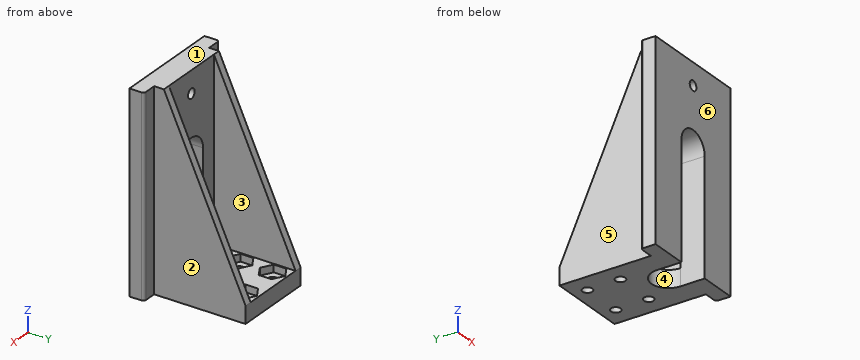
Autodesk Inventor part; units mm, degrees
ref_plane "YZ Plane" through (0, 0, 0) normal (1, 0, 0) x (0, 1, 0)
ref_plane "XZ Plane" through (0, 0, 0) normal (0, 1, 0) x (-1, 0, 0)
ref_plane "XY Plane" through (0, 0, 0) normal (0, 0, 1) x (1, 0, 0)
sketch "Sketch1" plane through (0, 0, 0) normal (0, 0, 1) x (1, 0, 0)
  line L0 (0, 43.4) -> (27, 43.4)
  line L1 (27, 43.4) -> (27, 0)
  line L2 (27, 0) -> (0, 0)
  line L3 (0, 0) -> (0, 43.4)
  circle A0 centre (5, 37.4) radius 2
  circle A1 centre (22, 37.4) radius 2
  circle A2 centre (5, 23.91) radius 2
  circle A3 centre (22, 23.91) radius 2
  dimension "d0" = 27
  dimension "d1" = 43.4
  dimension "d2" = 4
  dimension "d3" = 6
  dimension "d4" = 6
  dimension "d5" = 5
  dimension "d6" = 5
  dimension "d7" = 5
  dimension "d8" = 5
  dimension "d61" = 13.49
  dimension "d62" = 13.49
extrude "Extrusion1" add sketch "Sketch1" along normal blind 7
sketch "Sketch2" plane through (0, 0, 7) normal (0, 0, 1) x (1, 0, 0)
  line L0 (0, 10) -> (27, 10)
  line L1 (27, 10) -> (27, 0)
  line L2 (27, 0) -> (0, 0)
  line L3 (0, 0) -> (0, 10)
  line L4 (0, 0) -> (27, 0)
  line L5 (0, 43.4) -> (0, 0)
  line L6 (27, 0) -> (27, 43.4)
  dimension "d13" = 10
extrude "Extrusion2" add sketch "Sketch2" along normal blind 73
sketch "Sketch3" plane through (0, 0, 7) normal (0, 0, 1) x (1, 0, 0)
  line L0 (0.5, 39.9981) -> (0.5, 34.8019)
  line L1 (0.5, 34.8019) -> (5, 32.2038)
  line L2 (5, 32.2038) -> (9.5, 34.8019)
  line L3 (9.5, 34.8019) -> (9.5, 39.9981)
  line L4 (9.5, 39.9981) -> (5, 42.5962)
  line L5 (5, 42.5962) -> (0.5, 39.9981)
  circle A0 centre (5, 37.4) radius 4.5
  circle A1 centre (5, 37.4) radius 2
  line L6 (17.5, 39.9981) -> (17.5, 34.8019)
  line L7 (17.5, 34.8019) -> (22, 32.2038)
  line L8 (22, 32.2038) -> (26.5, 34.8019)
  line L9 (26.5, 34.8019) -> (26.5, 39.9981)
  line L10 (26.5, 39.9981) -> (22, 42.5962)
  line L11 (22, 42.5962) -> (17.5, 39.9981)
  circle A2 centre (22, 37.4) radius 4.5
  line L12 (17.5, 26.5081) -> (17.5, 21.3119)
  line L13 (17.5, 21.3119) -> (22, 18.7138)
  line L14 (22, 18.7138) -> (26.5, 21.3119)
  line L15 (26.5, 21.3119) -> (26.5, 26.5081)
  line L16 (26.5, 26.5081) -> (22, 29.1062)
  line L17 (22, 29.1062) -> (17.5, 26.5081)
  circle A3 centre (22, 23.91) radius 4.5
  line L18 (0.5, 26.5081) -> (0.5, 21.3119)
  line L19 (0.5, 21.3119) -> (5, 18.7138)
  line L20 (5, 18.7138) -> (9.5, 21.3119)
  line L21 (9.5, 21.3119) -> (9.5, 26.5081)
  line L22 (9.5, 26.5081) -> (5, 29.1062)
  line L23 (5, 29.1062) -> (0.5, 26.5081)
  circle A4 centre (5, 23.91) radius 4.5
  circle A5 centre (22, 37.4) radius 2
  circle A6 centre (22, 23.91) radius 2
  circle A7 centre (5, 23.91) radius 2
  point P0 (0, 0)
  dimension "d16" = 120
  dimension "d17" = 120
  dimension "d18" = 9
  dimension "d19" = 120
  dimension "d20" = 120
  dimension "d21" = 9
  dimension "d22" = 120
  dimension "d23" = 120
  dimension "d24" = 9
  dimension "d25" = 120
  dimension "d26" = 120
  dimension "d27" = 9
extrude "Extrusion3" cut sketch "Sketch3" against normal blind 3 contours L5 A0 L0 | A0 L1 L0 | A0 | L5 L4 A0 | A0 L2 L1 | L4 L3 A0 | A0 L3 L2 | A1 | L11 A2 L6 | A2 L7 L6 | A2 | L11 L10 A2 | A2 L8 L7 | L10 L9 A2 | A2 L9 L8 | L17 A3 L12 | A3 L13 L12 | A3 | L17 L16 A3 | A3 L14 L13 | L16 L15 A3 | A3 L15 L14 | L23 A4 L18 | A4 L19 L18 | A4 | L23 L22 A4 | A4 L20 L19 | L22 L21 A4 | A4 L21 L20 | A5 | A6 | A7
sketch "Sketch4" plane through (27, 0, 0) normal (1, 0, 0) x (0, 0, -1)
  line L0 (-80, 10) -> (-80, 0)
  line L1 (-7, 43.4) -> (-80, 10)
  line L2 (-80, 10) -> (-80, 0)
  line L3 (0, 43.4) -> (0, 0)
  line L4 (-80, 0) -> (0, 0)
  line L5 (0, 0) -> (0, 43.4)
  line L6 (0, 43.4) -> (-7, 43.4)
  line L7 (0, 43.4) -> (-7, 43.4)
extrude "Extrusion4" add sketch "Sketch4" along normal blind 3
sketch "Sketch5" plane through (0, 0, 0) normal (-1, 0, 0) x (0, 0, 1)
  line L0 (80, 0) -> (0, 0)
  line L1 (80, 10) -> (80, 0)
  line L2 (80, 0) -> (80, 10)
  line L3 (7, 43.4) -> (80, 10)
  line L4 (80, 10) -> (7, 43.4)
  line L5 (0, 43.4) -> (7, 43.4)
  line L6 (7, 43.4) -> (0, 43.4)
  line L7 (0, 43.4) -> (0, 0)
  line L8 (0, 43.4) -> (0, 0)
  line L9 (0, 0) -> (80, 0)
extrude "Extrusion5" add sketch "Sketch5" along normal blind 3
sketch "Sketch6" plane through (27, 10, 80) normal (0, 1, 0) x (1, 0, 0)
  circle A0 centre (-13.5, 9) radius 2
  line L0 (-27, 0) -> (-27, 73)
  line L1 (0, 0) -> (-27, 0)
  line L2 (-30, 80) -> (3, 80)
  point P0 (-27, 80)
  dimension "d34" = 4
  dimension "d35" = 13.5
  dimension "d45" = 71
extrude "Extrusion6" cut sketch "Sketch6" against normal blind 74
sketch "Sketch7" plane through (30, 0, 0) normal (0, -1, 0) x (1, 0, 0)
  line L0 (-9.5, 47) -> (-9.5, 0)
  line L1 (-9.5, 0) -> (-23.5, 0)
  line L2 (-23.5, 0) -> (-23.5, 47)
  line L3 (0, 80) -> (0, 0)
  line L4 (-33, 0) -> (-33, 80)
  line L5 (-33, 0) -> (0, 0)
  arc A0 (-9.5, 47) -> (-23.5, 47) centre (-16.5, 47) ccw
  point P0 (-30, 0)
  dimension "d39" = 33
  dimension "d40" = 14
  dimension "d41" = 9.5
  dimension "d42" = 47
extrude "Extrusion7" cut sketch "Sketch7" against normal blind 10
sketch "Sketch8" plane through (0, 0, 0) normal (0, 0, -1) x (-1, 0, 0)
  line L0 (-27, 10) -> (0, 10)
  circle A0 centre (-13.5, 10) radius 7
  point P0 (0, 0)
  point P1 (-6.5, 10)
  point P2 (-20.5, 10)
extrude "Extrusion8" cut sketch "Sketch8" against normal blind 74 contours A0 L0 picked at (-15.8333, 12.1687)
sketch "Sketch10" plane through (0, 0, 0) normal (0, 0, -1) x (-1, 0, 0)
  line L0 (3, 6) -> (9, 6)
  line L1 (9, 6) -> (9, 0)
  line L2 (9, 0) -> (3, 0)
  line L3 (3, 0) -> (3, 6)
  line L4 (3, 0) -> (-6.5, 0)
  line L5 (3, 43.4) -> (3, 0)
  line L6 (-36, 6) -> (-30, 6)
  line L7 (-30, 6) -> (-30, 0)
  line L8 (-30, 0) -> (-36, 0)
  line L9 (-36, 0) -> (-36, 6)
  point P0 (0, 0)
  point P1 (-30, 0)
  dimension "d56" = 6
  dimension "d57" = 6
extrude "Extrusion10" add sketch "Sketch10" against normal up to surface (80 mm away)
fillet "Fillet1" radius 1 2 edges at (-9, 6, 40) (36, 6, 40)
properties part number "1322_Clamp Holder_V1" material "Acetal Resin, White"
Build history of the part. All positions in model axes, mm. Face numbers are marked on the shaded views. A direction names the side the tool comes from. Give positions to 0.01 mm unless a question says otherwise; leave off trailing zeros. Loops run counter-clockwise (first coordinate to the right, second up) from the corner with the lowest first, then second, coordinate; pieces in that order, holes last.
1) Band-saw the part on C-C on y = 23.91. List the corners of the cut face in (x, z).
Values follow:
outline: (-3, 0) - (3, 0) - (3, 4) - (0.5, 4) - (0.5, 7) - (0, 7) - (0, 49.6) - (-3, 49.6) - close; (7, 0) - (20, 0) - (20, 4) - (17.5, 4) - (17.5, 7) - (9.5, 7) - (9.5, 4) - (7, 4) - close; (24, 0) - (30, 0) - (30, 49.6) - (27, 49.6) - (27, 7) - (26.5, 7) - (26.5, 4) - (24, 4) - close
2) Band-saw the part on A-A on x = 13.5. List the corners of the cut face in (y, z), then the cut area to 3 significant figures.
Values follow:
outline: (0, 54) - (10, 54) - (10, 69) - (0, 69) - close; (0, 73) - (10, 73) - (10, 80) - (0, 80) - close; (17, 0) - (43.4, 0) - (43.4, 7) - (17, 7) - close
area: 405 mm2
3) Band-saw the part on B-B on z = 15. List the corners of the cut face in (x, y), then the cut area to 3 significant figures.
Values follow:
outline: (-9, 0) - (6.5, 0) - (6.5, 10) - (0, 10) - (0, 39.74) - (-3, 39.74) - (-3, 6) - (-8, 6) arc R1 ccw to (-9, 5) - close; (20.5, 0) - (36, 0) - (36, 5) arc R1 ccw to (35, 6) - (30, 6) - (30, 39.74) - (27, 39.74) - (27, 10) - (20.5, 10) - close
area: 440 mm2
4) Band-saw the part on D-D on z = 50.5. List the corners of the cut face in (x, y).
Values follow:
outline: (-9, 0) - (7.44, 0) - (7.44, 10) - (0, 10) - (0, 23.5) - (-3, 23.5) - (-3, 6) - (-8, 6) arc R1 ccw to (-9, 5) - close; (19.56, 0) - (36, 0) - (36, 5) arc R1 ccw to (35, 6) - (30, 6) - (30, 23.5) - (27, 23.5) - (27, 10) - (19.56, 10) - close
5) Two-plate mould, pull along X, no slides. Class the marked faces 4, 5 and 6: released by +X, released by -X, zero draft, split by the parting line, or undercut.
Values follow:
face 4: undercut
face 5: released by -X
face 6: zero draft
6) Drop flat-ended pins along their axis: P1, Ø18.5, axis at y = 18.5, z = 23.5, coming from the -X side; P2, Ø3, axis at x = 28, z = 30.5, coming from the -Y side; P3, Ø7, axis at x = 22.5, y = 36, coming from the +Z side; P4, Ø8, axis at y = 20.5, z = 55.5, coming from the +X side. Give the stop position or say it passes through.
Values follow:
P1: stops at x = -3
P2: stops at y = 0
P3: stops at z = 7
P4: stops at x = 30
7) Probe line 1 along Y through (x, z) = (22, 2.2); line 2 along X through (y, z) = (8, 29); line 3 along X through (y, z) = (21, 19). List the from-to ranges inside material, lowest first.
Values follow:
line 1: y = 0 to 21.91, 25.91 to 35.4, 39.4 to 43.4
line 2: x = -3 to 6.5, 20.5 to 30
line 3: x = -3 to 0, 27 to 30
8) 3-axis set-ups, long thin cutter, end or side, ignore diameter. For the marked faces 1, 2 and 3: which of +Z, -Z, +X, -X, +Y, -Y reach the whole face in a straight line?
Values follow:
face 1: +Z, +X, -X, +Y, -Y
face 2: +Z, -Z, +X, +Y
face 3: +Z, +Y
